Design review of the part built by this model. Coordinates are the model's own, in mm. Face numbers are marked on the shaded views. A direction names the side the tool comes from. Round coordinates to 2 decimals unless told otherwise and drop trailing zeros. Loops run counter-clockwise (first coordinate to the right, second up) from the corner with the lowest first, then second, coordinate; pieces in that order, holes last. Notation, with made-up numbers: M 26.5,19.5 L 57.5,19.5 A22 cw 57.5,34.5 Z; hole C -24,22 d3. An arc over 180 degrees is marked long. Use a Markdown table: item, result.
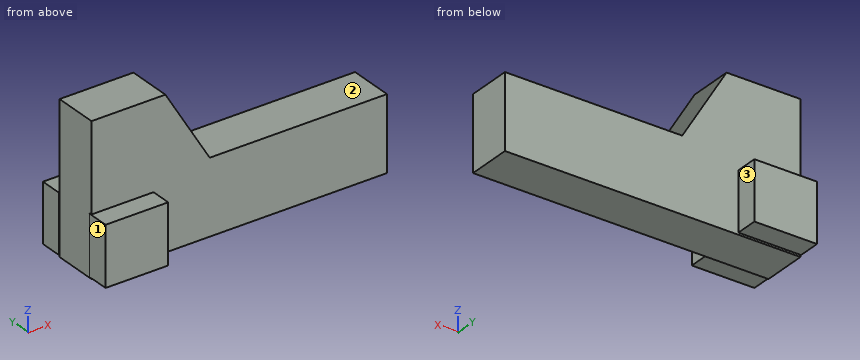
from build123d import *

# Parameters (mm, degrees)
F1_DEPTH = 19.05
F3_START = -44.45
F2_W     = 9.525
F2_H     = 25.4
F2_H_2   = 25.0668842345
F3_DEPTH = 26.924


with BuildPart() as f1:
    # F0 (on Front) → F1 (new body)
    with BuildSketch(Plane.XZ):
        Polygon((-71.1200013757, 17.3011439145), (-71.1200013757, -46.1988560855), (55.8799986243, -46.1988560855), (55.8799986243, -14.4488560855), (-20.3200013757, -14.4488560855), (-39.3700013757, 17.3011439145), align=None)
    extrude(amount=F1_DEPTH)

    # F2 (on Right) → F3 (join)
    with BuildSketch(Plane.YZ.offset(F3_START)):
        with Locations((-23.0265576392, -32.9159003079)):
            Rectangle(F2_W, F2_H)
        with Locations((4.7625, -32.7909840271)):
            Rectangle(F2_W, F2_H_2)
    extrude(amount=-F3_DEPTH)


solid = f1.part
1. Take a section at C-C on y = -25. Give the boundary of the cut face in (x, z).
Check values:
| item | result |
|---|---|
| outline | M -71.37,-45.62 L -44.45,-45.62 L -44.45,-20.22 L -71.37,-20.22 Z |
2. Insertion check: pin 1 (3 mm diameter, centred on y = 5.5, z = -30, fed in from +X); pin 2 (5 mm diameter, centred on x = 38, z = -14, fed in from -Y); pin 3 (3 mm diameter, centred on x = -57.5, y = 4, fed in from +Z); pin 4 (8 mm diameter, centred on x = 28, z = -8, fed in from -Y). Each pin has a flat end and moves straight along its axis. Give the tip position at first contact, or say it passes through.
Check values:
| item | result |
|---|---|
| pin 1 | stops at x = -44.45 |
| pin 2 | stops at y = -19.05 |
| pin 3 | stops at z = -20.26 |
| pin 4 | passes through |
3. Take a section at B-B on x = -55. Give the boundary of the cut face in (y, z) (3 decimals), and give its area (3 significant figures).
Check values:
| item | result |
|---|---|
| outline | M -27.789,-45.616 L -19.05,-45.616 L -19.05,-46.199 L 0,-46.199 L 0,-45.324 L 9.525,-45.324 L 9.525,-20.258 L 0,-20.258 L 0,17.301 L -19.05,17.301 L -19.05,-20.216 L -27.789,-20.216 Z |
| area | 1,670 mm² |
4. Take a section at D-D on y = -4. Give the boundary of the cut face in (x, z), and give its area (3 significant figures).
Check values:
| item | result |
|---|---|
| outline | M -71.12,-46.2 L 55.88,-46.2 L 55.88,-14.45 L -20.32,-14.45 L -39.37,17.3 L -71.12,17.3 Z |
| area | 5,340 mm² |
5. Machinability: for the marked faces 1, 2 and 3, which of the approach directions +Z, -Z, +X, -X, +Y, -Y give a long, thin tool a straight path to every point of the face, cutting with its end or side? Answer none if there is none.
Check values:
| item | result |
|---|---|
| face 1 | +Z, -Z, -X, +Y, -Y |
| face 2 | +Z, +X, +Y, -Y |
| face 3 | +Z, -Z, +X, +Y |
6. Wall thickness on line 1 along Y through (x, z) = (-64.5, -11); line 2 along Z through (x, y) = (2.5, -8); line 3 along X through (y, z) = (-4, -34.5): over which ranges is each line inside the solid? List them lowest first. Write a range as from..to.
Check values:
| item | result |
|---|---|
| line 1 | y = -19.05..0 |
| line 2 | z = -46.2..-14.45 |
| line 3 | x = -71.12..55.88 |
7. Take a section at A-A on z = -25.5. Give the boundary of the cut face in (x, y) (3 decimals).
Check values:
| item | result |
|---|---|
| outline | M -71.374,-27.789 L -44.45,-27.789 L -44.45,-19.05 L 55.88,-19.05 L 55.88,0 L -44.45,0 L -44.45,9.525 L -71.374,9.525 L -71.374,0 L -71.12,0 L -71.12,-18.264 L -71.374,-18.264 Z |
